```python
from build123d import *

# Parameters (mm, degrees)
F0_R      = 11.1
F1_DEPTH  = 3.5
F2_R      = 8.1
F4_DEPTH  = 1.65
F6_DEPTH  = 7.001
F7_R      = 3
F8_DEPTH  = 7.001
F9_R      = 3.875
F9_R_2    = 3
F10_DEPTH = 7


# Not quite as in the source:
# - a pattern or mirror of a feature is missing from the dataset's text; its kind, count and spacing are read off the source's solid


with BuildPart() as f1:
    # F0 (on Top) → F1 (new body, symmetric)
    with BuildSketch(Plane.XY):
        with BuildLine():
            ThreePointArc((40, 2), (36.7781745931, 9.7781745931), (29, 13))
            Line((29, 13), (-29, 13))
            ThreePointArc((-29, 13), (-36.7781745931, 9.7781745931), (-40, 2))
            Line((-40, 2), (-40, -2))
            ThreePointArc((-40, -2), (-36.7781745931, -9.7781745931), (-29, -13))
            Line((-29, -13), (29, -13))
            ThreePointArc((29, -13), (36.7781745931, -9.7781745931), (40, -2))
            Line((40, -2), (40, 2))
        make_face()
        Circle(F0_R, mode=Mode.SUBTRACT)
    extrude(amount=F1_DEPTH, both=True)

    # F2 (on Top) → F4 (cut, symmetric)
    with BuildSketch(Plane.XY):
        with Locations((-29.9, 0)):
            Circle(F2_R)
    f4 = extrude(amount=F4_DEPTH, both=True, mode=Mode.SUBTRACT)

    # F4_copies: F4 across plane
    add(f4.mirror(Plane(origin=(0, 0, 0), x_dir=(0, 0, 1), z_dir=(1, 0, 0))), mode=Mode.SUBTRACT)

    # F5 (on face) → F6 (cut, through all)
    with BuildSketch(Plane.XY.offset(3.5)):
        with BuildLine():
            ThreePointArc((-7.1140705647, -11), (-13.1, 0), (-7.1140705647, 11))
            Line((-7.1140705647, 11), (-28.4133931253, 11))
            ThreePointArc((-28.4133931253, 11), (-21.542029663, 7.3044049618), (-18.8, 0))
            ThreePointArc((-18.8, 0), (-21.542029663, -7.3044049618), (-28.4133931253, -11))
            Line((-28.4133931253, -11), (-7.1140705647, -11))
        make_face()
    f6 = extrude(amount=-F6_DEPTH, mode=Mode.SUBTRACT)

    # F6_copies: F6 across plane
    add(f6.mirror(Plane(origin=(0, 0, 0), x_dir=(0, 0, 1), z_dir=(1, 0, 0))), mode=Mode.SUBTRACT)

    # F7 (on face) → F8 (cut, through all)
    with BuildSketch(Plane.XY.offset(3.5)):
        with Locations((29.9, 0)):
            Circle(F7_R)
        with Locations((-29.9, 0)):
            Circle(F7_R)
    extrude(amount=-F8_DEPTH, mode=Mode.SUBTRACT)

    # F9 (on face) → F10 (join, through all)
    with BuildSketch(Plane.XY.offset(3.5)):
        with Locations((29.9, 0)):
            Circle(F9_R)
        with Locations((29.9, 0)):
            Circle(F9_R_2, mode=Mode.SUBTRACT)
    extrude(amount=-F10_DEPTH)


solid = f1.part
```
The model under review builds one solid part; all positions refer to its coordinate system, in mm. A direction names the side the tool comes from. Round coordinates to 2 decimals unless told otherwise and drop trailing zeros. Loops run counter-clockwise (first coordinate to the right, second up) from the corner with the lowest first, then second, coordinate; pieces in that order, holes last. Notation, with made-up numbers: (25, -27.5) -> (83, -27.5) arc R23 cw to (83, -2.5) -> close; hole circle Ø6 at (19, -9.5). An arc over 180 degrees is marked (long way). Answer as a JSON object with one key per item and string values. Group by question number.
1) We need section C-C on x = 29.9. Write out the cut boundary in (y, z) (3 decimals), then the cut area to 3 significant figures.
2) We need section B-B on y = -9.5. Write out the cut boundary in (x, z).
3) Mouldability with a two-part tool opening along X and no side actions: class faces 1 (the face through (-36.692, 9.863, 0.049)), 2 (the face through (-18, 11, 0)), 3 (the face through (-1, 12, 3.5)) as released by +X, released by -X, zero draft, split by the parting line, or undercut.
4) For pin 1 Ø2 at (y, z) = (-3.5, -2.5) entering from -X; pin 2 Ø2 at (y, z) = (-8.5, 0) entering from +X; pin 3 Ø3 at (y, z) = (-10.5, 0.5) entering from -X, all flat-tipped, find the tip position at first contact; note any pin that passes through.
5) For faces 4 (the face through (5.97, 9.36, -0.05)), 5 (the face through (38, 0, 0)), list the 3-axis set-ups (+Z, -Z, +X, -X, +Y, -Y) from which the entire face can be reached by the end or side of a thin tool; tool diameter is ignored.
6) We need section A-A on x = 0. Write out the cut boundary in (y, z), then the cut area to 3 significant figures.
7) For line 1 (X direction, y = -7.5, z = -0.5); line 2 (X direction, y = -7, z = -0.5); line 3 (X direction, y = -9.75, z = -0.75), list the stretches that pass through material, from the lowest coordinate up. Write a range as [from, to].
8) We need section D-D on x = -29.9. Write out the cut boundary in (y, z).
Result set:
{
 "1": {"outline": "(-12.963, -3.5) -> (-3, -3.5) -> (-3, 3.5) -> (-12.963, 3.5) -> close; (3, -3.5) -> (12.963, -3.5) -> (12.963, 3.5) -> (3, 3.5) -> close; hole (-8.1, -1.65) -> (-3.875, -1.65) -> (-3.875, 1.65) -> (-8.1, 1.65) -> close; hole (3.875, -1.65) -> (8.1, -1.65) -> (8.1, 1.65) -> (3.875, 1.65) -> close", "area": "112 mm²"},
 "2": {"outline": "(-37.05, -3.5) -> (-24.16, -3.5) -> (-24.16, 3.5) -> (-37.05, 3.5) -> close; (-9.02, -3.5) -> (-5.74, -3.5) -> (-5.74, 3.5) -> (-9.02, 3.5) -> close; (5.74, -3.5) -> (9.02, -3.5) -> (9.02, 3.5) -> (5.74, 3.5) -> close; (24.16, -3.5) -> (37.05, -3.5) -> (37.05, 3.5) -> (24.16, 3.5) -> close"},
 "3": {"face 1": "released by -X", "face 2": "undercut", "face 3": "zero draft"},
 "4": {"pin 1": "x = -39.99", "pin 2": "x = 38.53", "pin 3": "x = -37.49"},
 "5": {"face 4": "+Z, -Z", "face 5": "none"},
 "6": {"outline": "(-13, -3.5) -> (-11.1, -3.5) -> (-11.1, 3.5) -> (-13, 3.5) -> close; (11.1, -3.5) -> (13, -3.5) -> (13, 3.5) -> (11.1, 3.5) -> close", "area": "26.6 mm²"},
 "7": {"line 1": "[-38.53, -32.96], [-26.84, -21.72], [-10.74, -8.18], [8.18, 10.74], [21.72, 26.84], [32.96, 38.53]", "line 2": "[-38.8, -33.98], [-25.82, -21.29], [-11.07, -8.61], [8.61, 11.07], [21.29, 25.82], [33.98, 38.8]", "line 3": "[-36.81, -24.59], [-8.75, -5.31], [5.31, 8.75], [24.59, 36.81]"},
 "8": {"outline": "(-12.96, -3.5) -> (-3, -3.5) -> (-3, -1.65) -> (-8.1, -1.65) -> (-8.1, 1.65) -> (-3, 1.65) -> (-3, 3.5) -> (-12.96, 3.5) -> close; (3, -3.5) -> (12.96, -3.5) -> (12.96, 3.5) -> (3, 3.5) -> (3, 1.65) -> (8.1, 1.65) -> (8.1, -1.65) -> (3, -1.65) -> close"}
}
